Source: CAD feature listing. Evaluate the final solid. Frame: model axes, mm. A direction names the side the tool comes from. Give positions to 0.01 mm unless a question says otherwise; leave off trailing zeros. Order: outer loops, then holes, each group sorted by start corner. A loop starts at its lowest first (then second) coordinate and runs counter-clockwise, first axis right, second up.
1) Section C-C, the plane z = -6. Return loops of the section in (x, y), plus the area to 3 significant figures.
2) Access query for faces 4 (the face through (3.4, 1.01, 13.27)), 5 (the face through (0, 1, -12)). Directions: +Z, -Z, +X, -X, +Y, -Y. A direction counts if a zero-diameter tool reaches every point of the face in a straight line with its end or side. Return the directions, or none.
3) Section A-A, the plane z = 0. Return loops of the section in (x, y), plus the area to 3 significant figures.
4) Section B-B, the plane y = 0.7. Give the number of separate pieces and of enclosed holes in the cut face, plus the area to 3 significant figures.
5) First-contact query: P1, Ø1, axis at x = -9.5, y = 1, coming from the +Z side; P2, Ø1.4, axis at x = 8, z = -14.5, coming from the +Y side. Flat tips, straight axial feed; report the tip coordinate or a pass-through.
6) Material intervals for line 1 (Z direction, x = 0.5, y = 0.65); line 2 (X direction, y = 1.25, z = 0); line 3 (X direction, y = 1.1, z = -13.5), sorted ascending.
7) Draft query along X for faces 1 (the face through (11.75, 1.01, -11.91)), 2 (the face through (-7.95, 1.01, -15.65)), 3 (the face through (-3.364, 1.014, 13.31)). Return one class per face: released by +X, released by -X, zero draft, split by the parting line, or undercut.
```python
from build123d import *

# Parameters (mm, degrees)
SKETCH_1_W          = 24
SKETCH_1_H          = 24
EXTRUDE_1_DEPTH     = 2
SKETCH_2_R          = 1.15
EXTRUDE_2_DEPTH     = 2
FILLET_1_R          = 10
SKETCH_3_R          = 6.75
CUT_EXTRUDE_1_DEPTH = 2
FILLET_2_R          = 10


with BuildPart() as part:
    # Эскиз1 → Бобышка-Вытянуть1 (new body)
    with BuildSketch(Plane(origin=(0, 0, 0), x_dir=(1, 0, 0), z_dir=(0, 1, 0))):
        Rectangle(SKETCH_1_W, SKETCH_1_H)
    extrude(amount=EXTRUDE_1_DEPTH)

    # Эскиз2 → Бобышка-Вытянуть2 (add)
    # profile 1 of 3: a face of its own
    with BuildSketch(Plane(origin=(0, 2, 0), x_dir=(1, 0, 0), z_dir=(0, 1, 0))):
        with BuildLine():
            Line((-6.32455532, -12), (6.32455532, -12))
            ThreePointArc((6.32455532, -12), (3.843860629, -12.862141838), (2.432521277, -15.076923077))
            ThreePointArc((2.432521277, -15.076923077), (0, -17), (-2.432521277, -15.076923077))
            ThreePointArc((-2.432521277, -15.076923077), (-3.843860629, -12.862141838), (-6.32455532, -12))
        make_face()
        with Locations(Location((0, -14.5, 0), (0, 0, 270))):
            Circle(SKETCH_2_R, mode=Mode.SUBTRACT)
    # profile 2 of 3: a face of its own
    with BuildSketch(Plane(origin=(0, 2, 0), x_dir=(1, 0, 0), z_dir=(0, 1, 0))):
        with BuildLine():
            Line((-12, 12), (-10.247191011, 15.595505618))
            ThreePointArc((-10.247191011, 15.595505618), (-7.72464788, 16.984789973), (-5.567478723, 15.076923077))
            ThreePointArc((-5.567478723, 15.076923077), (-4.156139371, 12.862141838), (-1.67544468, 12))
            Line((-1.67544468, 12), (-12, 12))
        make_face()
        with Locations(Location((-8, 14.5, 0), (0, 0, 270))):
            Circle(SKETCH_2_R, mode=Mode.SUBTRACT)
    # profile 3 of 3: a face of its own
    with BuildSketch(Plane(origin=(0, 2, 0), x_dir=(1, 0, 0), z_dir=(0, 1, 0))):
        with BuildLine():
            Line((12, 12), (1.67544468, 12))
            ThreePointArc((1.67544468, 12), (4.156139371, 12.862141838), (5.567478723, 15.076923077))
            ThreePointArc((5.567478723, 15.076923077), (7.72464788, 16.984789973), (10.247191011, 15.595505618))
            Line((10.247191011, 15.595505618), (12, 12))
        make_face()
        with Locations(Location((8, 14.5, 0), (0, 0, 90))):
            Circle(SKETCH_2_R, mode=Mode.SUBTRACT)
    extrude(amount=-EXTRUDE_2_DEPTH)

    # Скругление1
    fillet_1_edges = [part.edges().sort_by_distance(p)[0] for p in [
        (12, 1, 12),
        (-12, 1, 12),
    ]]
    fillet(fillet_1_edges, radius=FILLET_1_R)

    # Эскиз3 → Вырез-Вытянуть1 (cut)
    with BuildSketch(Plane(origin=(0, 2, 0), x_dir=(1, 0, 0), z_dir=(0, 1, 0))):
        with Locations(Location((0, 0, 0), (0, 0, 270))):
            Circle(SKETCH_3_R)
    extrude(amount=-CUT_EXTRUDE_1_DEPTH, mode=Mode.SUBTRACT)

    # Скругление2
    fillet_2_edges = [part.edges().sort_by_distance(p)[0] for p in [
        (-12, 1, -12),
        (12, 1, -12),
    ]]
    fillet(fillet_2_edges, radius=FILLET_2_R)


solid = part.part
```
From the geometry:
1. outline: (-12, 0) - (-3.09, 0) - (-3.09, 2) - (-12, 2) - close; (3.09, 0) - (12, 0) - (12, 2) - (3.09, 2) - close
1. area: 35.6 mm2
2. face 4: +Z, +X, +Y, -Y
2. face 5: -Z, +Y, -Y
3. outline: (-12, 0) - (-6.75, 0) - (-6.75, 2) - (-12, 2) - close; (6.75, 0) - (12, 0) - (12, 2) - (6.75, 2) - close
3. area: 21.0 mm2
4. separate pieces: 1
4. enclosed holes: 4
4. area: 470 mm2
5. P1: stops at z = 9.83
5. P2: passes through
6. line 1: z = -12 to -6.73, 6.73 to 13.46, 15.54 to 16.95
6. line 2: x = -12 to -6.75, 6.75 to 12
6. line 3: x = -11.25 to -8.57, -7.43 to -4.8, 4.8 to 7.43, 8.57 to 11.25
7. face 1: released by +X
7. face 2: undercut
7. face 3: released by -X
